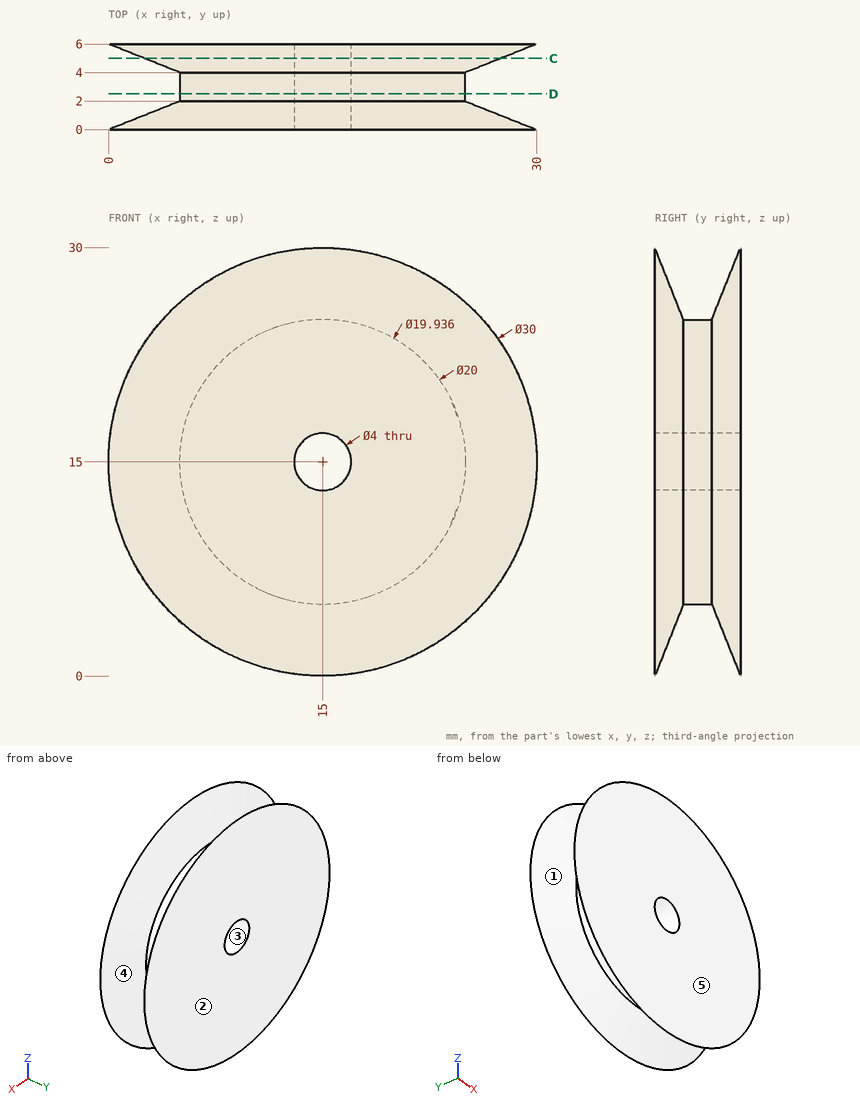
Job drawing, mm, ordinate dimensions from the low corner. One solid piece. A direction names the side the tool comes from. Round coordinates to 2 decimals unless told otherwise and drop trailing zeros. Loops run counter-clockwise (first coordinate to the right, second up) from the corner with the lowest first, then second, coordinate; pieces in that order, holes last.
(1) Cut at D-D (y = 2.5). Give the cut face in (x, z), plus the area to 3 significant figures.
(2) Which spindle directions (+Z, -Z, +X, -X, +Y, -Y) get a long thin tool onto all of the face, cutting with end or side? Do the marked faces 1 and 2. Say none if no direction does.
(3) Drop flat-ended pins along their axis: pin 1 (3 mm diameter, centred on x = 26.5, y = 1, fed in from +Z) (1 decimal); pin 2 (1.5 mm diameter, centred on x = 9.5, y = 0.5, fed in from +Z). Give the stop position or say it passes through.
(4) Cut at C-C (y = 5). Give the cut face in (x, z).
(5) Wall check: line 1 along Z through (x, y) = (15, 3); line 2 along Y through (x, z) = (24.75, 11.5) (1 decimal); line 3 along Y through (x, z) = (23.25, 21). Give the ranges that are in metal, low to high.
(6) Two-plate mould, pull along X, no slides. Class the marked faces 3, 4 and 5: +X half, -X half, draft (parallel to the pull), parting line (faces both ways), or undercut.
Findings below:
1. outline: circle Ø19.94 at (15, 15); hole circle Ø4 at (15, 15)
1. area: 300 mm2
2. face 1: none
2. face 2: +Z, -Z, +X, -X, +Y
3. pin 1: stops at z = 25.8
3. pin 2: stops at z = 29.16
4. outline: circle Ø25 at (15, 15); hole circle Ø4 at (15, 15)
5. line 1: z = 5.03 to 13, 17 to 24.97
5. line 2: y = 0 to 1.8, 4.1 to 6
5. line 3: y = 0 to 1.91, 4.08 to 6
6. face 3: undercut
6. face 4: parting line
6. face 5: draft
